```python
from build123d import *

# Parameters (mm, degrees)
SKETCH1_R             = 7.5
SKETCH1_R_2           = 5
BOSS_EXTRUDE1_DEPTH   = 3
SKETCH1_R_3           = 10
BOSS_EXTRUDE1_2_DEPTH = 3
SKETCH1_R_4           = 7
BOSS_EXTRUDE1_3_DEPTH = 3
SKETCH3_R             = 7
SKETCH3_R_2           = 7.5
SKETCH3_R_3           = 10
BOSS_EXTRUDE2_DEPTH   = 27
BOSS_EXTRUDE3_DEPTH   = 3
SKETCH5_R             = 2.5
CUT_EXTRUDE1_DEPTH    = 34


with BuildPart() as part:
    # Sketch1 → Boss-Extrude1 (new body)
    with BuildSketch(Plane.XY):
        with Locations((29, 78)):
            Circle(SKETCH1_R)
        with Locations((29, 78)):
            Circle(SKETCH1_R_2, mode=Mode.SUBTRACT)
    extrude(amount=BOSS_EXTRUDE1_DEPTH)



with BuildPart() as body_2:
    # Sketch1 → Boss-Extrude1 2 (new body)
    with BuildSketch(Plane.XY):
        with Locations((-9.3, 45)):
            Circle(SKETCH1_R_3)
        with Locations((-9.3, 45)):
            Circle(SKETCH1_R_2, mode=Mode.SUBTRACT)
    extrude(amount=BOSS_EXTRUDE1_2_DEPTH)


with BuildPart() as body_3:
    # Sketch1 → Boss-Extrude1 3 (new body)
    with BuildSketch(Plane.XY):
        with Locations((29, 12)):
            Circle(SKETCH1_R_4)
        with Locations((29, 12)):
            Circle(SKETCH1_R_2, mode=Mode.SUBTRACT)
    extrude(amount=BOSS_EXTRUDE1_3_DEPTH)


with BuildPart() as part_1:
    add(part.part)

    add(body_2.part)  # Boss-Extrude2 merges body 2

    add(body_3.part)  # Boss-Extrude2 merges body 3
    # Sketch3 → Boss-Extrude2 (add)
    with BuildSketch(Plane.XY.offset(3)):
        with Locations((29, 12)):
            Circle(SKETCH3_R)
        with Locations((29, 78)):
            Circle(SKETCH3_R_2)
        with Locations((-9.3, 45)):
            Circle(SKETCH3_R_3)
    extrude(amount=BOSS_EXTRUDE2_DEPTH)

    # Sketch4 → Boss-Extrude3 (add)
    with BuildSketch(Plane.XY.offset(30)):
        with BuildLine():
            ThreePointArc((-11.409189276, 35.22496442), (73.534073318, 45), (-11.409189276, 54.77503558))
            ThreePointArc((-11.409189276, 54.77503558), (-19.3, 45), (-11.409189276, 35.22496442))
        make_face()
    extrude(amount=BOSS_EXTRUDE3_DEPTH)

    # Sketch5 → Cut-Extrude1 (cut, through all)
    with BuildSketch(Plane.XY.offset(33)):
        with Locations((-9.3, 45)):
            Circle(SKETCH5_R)
        with Locations((29, 12)):
            Circle(SKETCH5_R)
        with Locations((29, 78)):
            Circle(SKETCH5_R)
    extrude(amount=-CUT_EXTRUDE1_DEPTH, mode=Mode.SUBTRACT)


solid = part_1.part
```
Check sheet for the modelled part. Datum: model origin and axes. Units: mm. A direction names the side the tool comes from. Give positions to 0.01 mm unless a question says otherwise; leave off trailing zeros. Order: outer loops, then holes, each group sorted by start corner. A loop starts at its lowest first (then second) coordinate and runs counter-clockwise, first axis right, second up. Notation, with made-up numbers: M 67.5,20 L 72.5,20 A22 cw 72.5,33 Z; hole C 51.25,72.25 d11. An arc over 180 degrees is marked long. Answer in a Markdown table with one row per item. Add a question column.
Q1. Gauge pin test, flat ends, axial feed: pin 1 Ø4.5 at (x, y) = (-9.3, 45) entering from -Z; pin 2 Ø3 at (x, y) = (8.5, 72.5) entering from -Z; pin 3 Ø1.5 at (y, z) = (51, 15.5) entering from +X; pin 4 Ø1 at (y, z) = (36, 10) entering from -X. Record the tip position at first contact, or that the pin passes through.
Q2. Sectioned sample at A-A, the plane z = 19. Record the boundary of the cut face in (x, y), and give its area (3 significant figures).
Q3. Release check for a two-part mould opening along X. For faces 3 (the flat face through (34, 76, 0)), 4 (the cylindrical face through (35.466, 9.319, 14.79)), 5 (the cylindrical face through (26.5, 78.1, 18.2)) record: released by +X, released by -X, zero draft, split by the parting line, or undercut.
Q4. Thickness scan on L1, parallel to Y at x = 29, z = 2.3; L2, parallel to Y at x = -9, z = 2; L3, parallel to Y at x = 28, z = 6.5. Record the ranges inside material, lowest first.
Q5. Sectioned sample at C-C, the plane x = 29. Record the boundary of the cut face in (y, z), and give its area (3 significant figures).
Q6. Sectioned sample at D-D, the plane x = -5.5. Record the boundary of the cut face in (y, z).
Q7. Access from +Z, -Z, +X, -X, +Y, -Y to the whole of each face (thin tool, end or side, straight path). Record for faces 1 (the cylindrical face through (24, 12, 1)), 2 (the cylindrical face through (-9.84, 42.56, 18.21)).
Q8. Sectioned sample at B-B, the plane y = 78. Record the boundary of the cut face in (x, z).
Verdict:
| question | item | result |
|---|---|---|
| 1 | pin 1 | through |
| 1 | pin 2 | z = 30 |
| 1 | pin 3 | x = -0.79 |
| 1 | pin 4 | x = -14.57 |
| 2 | outline | C -9.3,45 d20; C 29,78 d15; C 29,12 d14; hole C -9.3,45 d5; hole C 29,12 d5; hole C 29,78 d5 |
| 2 | area | 586 mm² |
| 3 | face 3 | zero draft |
| 3 | face 4 | split by the parting line |
| 3 | face 5 | undercut |
| 4 | L1 | 5 to 7, 17 to 19, 70.5 to 73, 83 to 85.5 |
| 4 | L2 | 35 to 40.01, 49.99 to 55 |
| 4 | L3 | 5.07 to 9.71, 14.29 to 18.93, 70.57 to 75.71, 80.29 to 85.43 |
| 5 | outline | M 1.99,30 L 5,30 L 5,0 L 7,0 L 7,3 L 9.5,3 L 9.5,33 L 1.99,33 Z; M 14.5,3 L 17,3 L 17,0 L 19,0 L 19,30 L 70.5,30 L 70.5,0 L 73,0 L 73,3 L 75.5,3 L 75.5,33 L 14.5,33 Z; M 80.5,3 L 83,3 L 83,0 L 85.5,0 L 85.5,30 L 88.01,30 L 88.01,33 L 80.5,33 Z |
| 5 | area | 768 mm² |
| 6 | outline | M 21.42,30 L 35.75,30 L 35.75,0 L 41.75,0 L 41.75,3 L 48.25,3 L 48.25,0 L 54.25,0 L 54.25,30 L 68.58,30 L 68.58,33 L 21.42,33 Z |
| 7 | face 1 | -Z |
| 7 | face 2 | +Z, -Z |
| 8 | outline | M 2.88,30 L 21.5,30 L 21.5,0 L 24,0 L 24,3 L 26.5,3 L 26.5,33 L 2.88,33 Z; M 31.5,3 L 34,3 L 34,0 L 36.5,0 L 36.5,30 L 58.12,30 L 58.12,33 L 31.5,33 Z |
